Autodesk Inventor part; units mm, degrees
ref_plane "YZ Plane" through (0, 0, 0) normal (1, 0, 0) x (0, 1, 0)
ref_plane "XZ Plane" through (0, 0, 0) normal (0, 1, 0) x (-1, 0, 0)
ref_plane "XY Plane" through (0, 0, 0) normal (0, 0, 1) x (1, 0, 0)
sketch "Sketch1" plane through (0, 0, 0) normal (0, 0, 1) x (1, 0, 0)
  line L0 (0, 0) -> (50.8, 0)
  line L1 (50.8, 0) -> (50.8, 12.7)
  line L2 (50.8, 12.7) -> (0, 12.7)
  line L3 (0, 12.7) -> (0, 0)
  dimension "d0" = 50.8
  dimension "d1" = 12.7
extrude "Extrusion1" add sketch "Sketch1" along normal blind 25.4
sketch "Sketch2" plane through (0, 0, 25.4) normal (0, 0, 1) x (1, 0, 0)
  line L0 (50.8, 12.7) -> (0, 12.7) construction
  line L1 (50.8, 0) -> (50.8, 12.7) construction
  line L2 (0, 12.7) -> (50.8, 12.7) construction
  line L3 (50.8, 12.7) -> (50.8, 6.35) construction
  line L4 (50.8, 6.35) -> (0, 6.35) construction
  line L5 (0, 6.35) -> (0, 12.7) construction
  point P0 (0, 0)
  point P1 (25.4, 6.35)
  point P2 (6.35, 6.35)
  point P3 (44.45, 6.35)
  dimension "d4" = 6.35
  dimension "d5" = 19.05
  dimension "d6" = 19.05
hole "Hole1" at (25.4, 6.35, 25.4) at (6.35, 6.35, 25.4) at (44.45, 6.35, 25.4) direction (0, 0, -1) diameter 5.1054 end through all
sketch "Sketch3" plane through (0, 0, 0) normal (-1, 0, 0) x (0, 0, 1)
  line L0 (0, 0) -> (0, 12.7)
  line L1 (0, 12.7) -> (25.4, 12.7)
  line L2 (0, 0) -> (25.4, 0)
  line L3 (25.4, 0) -> (25.4, 12.7)
  line L4 (25.4, 12.7) -> (0, 12.7)
  line L5 (0, 12.7) -> (0, 0)
extrude "Extrusion2" add sketch "Sketch3" along normal blind 76.2
sketch "Sketch4" plane through (50.8, 12.7, 25.4) normal (0, 1, 0) x (1, 0, 0)
  line L0 (-127, 25.4) -> (-127, 0)
  line L1 (-127, 12.7) -> (-134.3323, 12.7)
  line L2 (-134.3323, 12.7) -> (-127, 0)
  line L3 (-127, 0) -> (-127, 25.4)
  line L4 (-127, 25.4) -> (-134.3323, 12.7)
  point P0 (-50.8, 25.4)
  dimension "d16" = 7.3323
extrude "Extrusion3" add sketch "Sketch4" against normal up to surface (12.7 mm away)
sketch "Sketch5" plane through (50.8, 12.7, 25.4) normal (0, 1, 0) x (1, 0, 0)
  line L0 (-134.3323, 12.7) -> (-127, 0)
  line L1 (-127, 25.4) -> (-134.3323, 12.7)
  line L2 (0, 25.4) -> (-127, 25.4)
  line L3 (0, 0) -> (-127, 0)
  line L4 (0, 25.4) -> (0, 0)
  line L5 (-125.1669, 22.225) -> (-130.6662, 12.7)
  line L6 (-130.6662, 12.7) -> (-125.1669, 3.175)
  line L7 (-125.1669, 3.175) -> (-50.8, 3.175)
  line L8 (-50.8, 3.175) -> (-50.8, 22.225)
  line L9 (-50.8, 22.225) -> (-125.1669, 22.225)
  point P0 (-50.8, 25.4)
  dimension "d19" = 3.175
  dimension "d20" = 3.175
  dimension "d21" = 3.175
  dimension "d22" = 3.175
  dimension "d23" = 3.175
  dimension "d24" = 3.175
  dimension "d25" = 3.175
  dimension "d26" = 3.175
  dimension "d27" = 50.8
  dimension "d28" = 50.8
extrude "Extrusion4" cut sketch "Sketch5" against normal through all contours L9 L8 L7 L6 L5
sketch "Sketch6" plane through (0, 0, 0) normal (0, 0, 1) x (1, 0, 0)
  line L0 (-76.2, 0) -> (-76.2, 12.7) construction
  line L1 (-76.2, 6.35) -> (50.8, 6.35) construction
  line L2 (50.8, 0) -> (50.8, 12.7) construction
  point P0 (0, 0)
  point P1 (-57.15, 6.35)
  point P2 (-25.4, 6.35)
  dimension "d31" = 31.75
  dimension "d32" = 19.05
hole "Hole2" at (-57.15, 6.35, 0) at (-25.4, 6.35, 0) direction (0, 0, 1) diameter 5.1054 depth 8.89
sketch "Sketch7" plane through (0, 0, 25.4) normal (0, 0, 1) x (1, 0, 0)
  line L0 (-76.2, 0) -> (-76.2, 12.7) construction
  line L1 (-76.2, 6.35) -> (50.8, 6.35) construction
  line L2 (50.8, 0) -> (50.8, 12.7) construction
  point P0 (0, 0)
  point P1 (-38.1, 6.35)
  dimension "d40" = 38.1
hole "Hole3" at (-38.1, 6.35, 25.4) direction (0, 0, -1) diameter 5.1054 depth 16.51
fillet "Fillet1" radius 3.175 5 edges at (0, 6.35, 3.175) (0, 6.35, 22.225) (-74.3669, 6.35, 3.175) (-79.8662, 6.35, 12.7) (-74.3669, 6.35, 22.225)
chamfer "Chamfer1" [suppressed]
properties part number "Third Baseplate Spacer"
The model under review builds one solid part; all positions refer to its coordinate system, in mm. A direction names the side the tool comes from. Round coordinates to 2 decimals unless told otherwise and drop trailing zeros. Order: outer loops, then holes, each group sorted by start corner. A loop starts at its lowest first (then second) coordinate and runs counter-clockwise, first axis right, second up. Notation, with made-up numbers: (29, -30.75) - (34, -30.75) arc R26 ccw to (34, -4.75) - close; hole circle Ø6 at (-34.75, -37). An arc over 180 degrees is marked (long way). Use one line per item in the form item = value.
Q1. Add section C-C on x = -38.1. Give the boundary of the cut face in (y, z) (3 decimals).
Response values:
outline = (0, 0) - (12.7, 0) - (12.7, 3.175) - (0, 3.175) - close; (0, 22.225) - (3.797, 22.225) - (3.797, 25.4) - (0, 25.4) - close; (8.903, 22.225) - (12.7, 22.225) - (12.7, 25.4) - (8.903, 25.4) - close
Q2. Clearance check with flat-ended pins moving along their axes: P1, Ø1.5, axis at y = 6, z = 21.5, coming from the -X side; P2, Ø4, axis at x = -62, z = 21.5, coming from the -Y side; P3, Ø5, axis at y = 9.5, z = 16.5, coming from the -X side; P4, Ø4, axis at y = 5.5, z = 10, coming from the -X side. State where each tip first meets the part, or that it passes through.
Response values:
P1 = -78.88
P2 = 0
P3 = -82.78
P4 = -83.13
Q3. Mouldability with a two-part tool opening along X and no side actions: class faces 1 (the flat face through (-12, 6, 0)), 2 (the cylindrical face through (-74.14, 6.26, 3.61)), 3 (the flat face through (50.8, 6, 13)) as pulls with the +X half, pulls with the -X half, needs draft (parallel to the pull), parting line crosses it, or undercut.
Response values:
face_1 = needs draft
face_2 = undercut
face_3 = pulls with the +X half
Q4. Add section D-D on x = 6.35. Give the boundary of the cut face in (y, z).
Response values:
outline = (0, 0) - (3.8, 0) - (3.8, 25.4) - (0, 25.4) - close; (8.9, 0) - (12.7, 0) - (12.7, 25.4) - (8.9, 25.4) - close
Q5. Tool access review of faces 4 (the cylindrical face through (-59.68, 6.02, 1.61)), 5 (the flat face through (-0.5, 0, 4.1)), 6 (the flat face through (-77.09, 6.44, 7.89)): name each direction out of +Z, -Z, +X, -X, +Y, -Y from which nothing blocks a thin tool from reaching the whole face with its end or side.
Response values:
face_4 = -Z
face_5 = +Z, -Z, +X, -X, -Y
face_6 = +Y, -Y
Q6. To check wall thickness, follow line 1 (Z direction, x = -40.5, y = 8.75) (3 decimals); line 2 (X direction, y = 6.35, z = 1.3); line 3 (Y direction, x = -57.15, z = 2.1). State the ranges of each line that lie inside material, in increasing order.
Response values:
line_1 = 0 to 3.175, 22.225 to 25.4
line_2 = -76.95 to -59.7, -54.6 to -27.95, -22.85 to 3.8, 8.9 to 22.85, 27.95 to 41.9, 47 to 50.8
line_3 = 0 to 3.8, 8.9 to 12.7
Q7. Add section B-B on x = -65.5. Give the boundary of the cut face in (y, z) (3 decimals).
Response values:
outline = (0, 0) - (12.7, 0) - (12.7, 3.175) - (0, 3.175) - close; (0, 22.225) - (12.7, 22.225) - (12.7, 25.4) - (0, 25.4) - close
